Work out the finished part from the listing and answer in its coordinate system (mm). Face numbers are marked on the shaded views. A direction names the side the tool comes from. Coordinates: 2 decimals unless noted, no trailing zeros. Loops run counter-clockwise (first coordinate to the right, second up) from the corner with the lowest first, then second, coordinate; pieces in that order, holes last. Notation, with made-up numbers: (66, 18.25) -> (74, 18.25) arc R13 cw to (74, 36.25) -> close; hole circle Ø5 at (55, -23). An arc over 180 degrees is marked (long way). Use a Markdown table: item, result.
from build123d import *

# Parameters (mm, degrees)
SKETCH1_W           = 35
SKETCH1_H           = 25
BOSS_EXTRUDE1_DEPTH = 10
SKETCH2_R           = 3
CUT_EXTRUDE1_DEPTH  = 24.717082451
SKETCH3_W           = 18
SKETCH3_H           = 10
BOSS_EXTRUDE2_DEPTH = 20
SKETCH4_R           = 3
CUT_EXTRUDE2_DEPTH  = 38.831864876
FILLET2_R           = 15
FILLET3_R           = 2
CUT_EXTRUDE3_START  = -10
SKETCH5_R           = 3
CUT_EXTRUDE3_DEPTH  = 27.912057737
CUT_EXTRUDE4_START  = -10
CUT_EXTRUDE4_DEPTH  = 33.793107029


# Some blends are built 0.0001 mm under size
with BuildPart() as part:
    # Sketch1 → Boss-Extrude1 (new body)
    with BuildSketch(Plane.XY):
        Rectangle(SKETCH1_W, SKETCH1_H)
    extrude(amount=BOSS_EXTRUDE1_DEPTH)

    # Sketch2 → Cut-Extrude1 (cut, through all)
    with BuildSketch(Plane.XY.offset(10)):
        with Locations((-7.5, 2.5)):
            Circle(SKETCH2_R)
    extrude(amount=-CUT_EXTRUDE1_DEPTH, mode=Mode.SUBTRACT)

    # Sketch3 → Boss-Extrude2 (add)
    with BuildSketch(Plane.XY.offset(10)):
        with Locations((8.5, -7.5)):
            Rectangle(SKETCH3_W, SKETCH3_H)
    extrude(amount=BOSS_EXTRUDE2_DEPTH)

    # Sketch4 → Cut-Extrude2 (cut, through all)
    with BuildSketch(Plane(origin=(0, -2.5, 0), x_dir=(1, 0, 0), z_dir=(0, 1, 0))):
        with Locations(Location((8.5, -20, 0), (0, 0, 180))):
            Circle(SKETCH4_R)
    extrude(amount=-CUT_EXTRUDE2_DEPTH, mode=Mode.SUBTRACT)

    # Fillet2
    # the kernel refuses this fillet: 15 mm, written as the material it adds along each edge
    with BuildSketch(Plane(origin=(-0.5, -12.5, 10), x_dir=(-1, 0, 0), z_dir=(0, 1, 0))) as fillet2_piece_1:
        with BuildLine():
            CenterArc((FILLET2_R, FILLET2_R), FILLET2_R, 180, 90)
            Line((0, FILLET2_R), (0, 0))
            Line((0, 0), (FILLET2_R, 0))
        make_face()
    extrude(amount=10)
    with BuildSketch(Plane(origin=(-0.5, -2.5, 10), x_dir=(0, 1, 0), z_dir=(1, 0, 0))) as fillet2_piece_2_section:
        with BuildLine():
            CenterArc((FILLET2_R, FILLET2_R), FILLET2_R, 180, 90)
            Line((0, FILLET2_R), (0, 0))
            Line((0, 0), (FILLET2_R, 0))
        make_face()
    fillet2_piece_2 = extrude(amount=18, mode=Mode.PRIVATE)
    fillet2_piece_2 = fillet2_piece_2 - Plane(origin=(8.5, 1.000391612, 20), x_dir=(-1, 0, 0), z_dir=(0, 1, 0)) * Cylinder(3, 96, mode=Mode.PRIVATE)
    add(fillet2_piece_2)
    with BuildSketch(Plane(origin=(-0.5, -12.5, 10), x_dir=(-1, 0, 0), z_dir=(0, 1, 0))) as fillet2_piece_3a_section:
        with BuildLine():
            CenterArc((FILLET2_R, FILLET2_R), FILLET2_R, 180, 90)
            Line((0, FILLET2_R), (0, 0))
            Line((0, 0), (FILLET2_R, 0))
        make_face()
    fillet2_piece_3a = extrude(amount=47.5, mode=Mode.PRIVATE)
    fillet2_piece_3a = split(fillet2_piece_3a, bisect_by=Plane(origin=(-3.591955578, 12.5, 13.608814387), z_dir=(0, -1, 0)), keep=Keep.TOP, mode=Mode.PRIVATE)
    fillet2_piece_3a = fillet2_piece_3a - Plane(origin=(-7.5, 2.5, 13.608814387), x_dir=(1, 0, 0), z_dir=(0, 0, 1)) * Cylinder(3, 155, mode=Mode.PRIVATE)
    fillet2_piece_3a = split(fillet2_piece_3a, bisect_by=Plane(origin=(-3.591955578, -2.5, 13.608814387), z_dir=(0, 1, 0)), keep=Keep.TOP, mode=Mode.PRIVATE)
    with BuildSketch(Plane(origin=(-38, -2.5, 10), x_dir=(0, 1, 0), z_dir=(1, 0, 0))) as fillet2_piece_3b_section:
        with BuildLine():
            CenterArc((FILLET2_R, FILLET2_R), FILLET2_R, 180, 90)
            Line((0, FILLET2_R), (0, 0))
            Line((0, 0), (FILLET2_R, 0))
        make_face()
    fillet2_piece_3b = extrude(amount=55.5, mode=Mode.PRIVATE)
    fillet2_piece_3b = split(fillet2_piece_3b, bisect_by=Plane(origin=(-17.5, 8.593163462, 10.419487544), z_dir=(1, 0, 0)), keep=Keep.TOP, mode=Mode.PRIVATE)
    fillet2_piece_3b = fillet2_piece_3b - Plane(origin=(-7.5, 2.5, 10.419487544), x_dir=(1, 0, 0), z_dir=(0, 0, 1)) * Cylinder(3, 171, mode=Mode.PRIVATE)
    fillet2_piece_3b = split(fillet2_piece_3b, bisect_by=Plane(origin=(-0.5, 8.593163462, 10.419487544), z_dir=(-1, 0, 0)), keep=Keep.TOP, mode=Mode.PRIVATE)
    fillet2_piece_3 = fillet2_piece_3a & fillet2_piece_3b
    add(fillet2_piece_3)

    # Fillet3
    fillet3_edges = [part.edges().sort_by_distance(p)[0] for p in [
        (17.5, 0, 0),
        (-17.5, 0, 0),
        (-17.5, 0, 10),
        (-0.5, -7.5, 30),
        (17.5, -7.5, 30),
    ]]
    fillet(fillet3_edges, radius=FILLET3_R - 0.0001)  # a hair under: the kernel refuses the full size

    # Sketch5 → Cut-Extrude3 (cut, through all)
    with BuildSketch(Plane(origin=(0, 0, 0), x_dir=(-1, 0, 0), z_dir=(0, 0, -1)).offset(CUT_EXTRUDE3_START)):
        Polygon((2.5, 5.386751346), (2.5, -0.386751346), (7.5, -3.273502692), (12.5, -0.386751346), (12.5, 5.386751346), (7.5, 8.273502692), align=None)
        with Locations(Location((7.5, 2.5, 0), (0, 0, 180))):
            Circle(SKETCH5_R, mode=Mode.SUBTRACT)
    extrude(amount=-CUT_EXTRUDE3_DEPTH, mode=Mode.SUBTRACT)

    # Sketch6 → Cut-Extrude4 (cut, through all)
    with BuildSketch(Plane.XZ.offset(12.5).offset(CUT_EXTRUDE4_START)):
        Polygon((8.5, 14.111027254), (13.6, 17.055513627), (13.6, 22.944486373), (8.5, 25.888972746), (3.4, 22.944486373), (3.4, 17.055513627), align=None)
    extrude(amount=-CUT_EXTRUDE4_DEPTH, mode=Mode.SUBTRACT)


solid = part.part
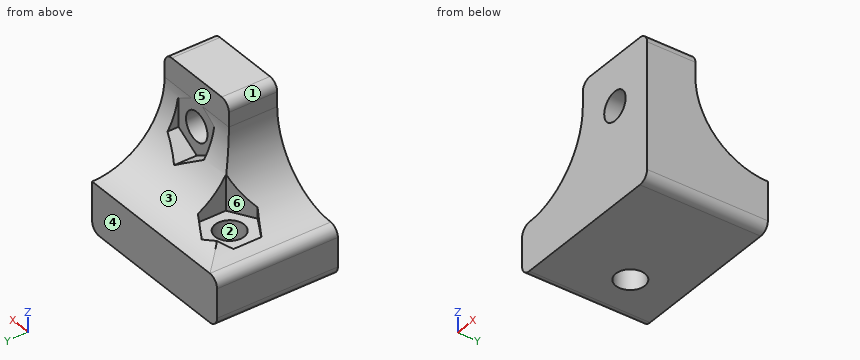
Q1. Determine the mould class of the marked faces 1, 2 and 3 for opening direction Y: pulls with the +Y half, pulls with the -Y half, needs draft (parallel to the pull), parting line crosses it, or undercut.
Solved:
| item | result |
|---|---|
| face 1 | needs draft |
| face 2 | undercut |
| face 3 | pulls with the +Y half |
Q2. For the marked faces 4, 5 and 6, determine the directions among +Z, -Z, +X, -X, +Y, -Y from which every point of the face is accessible in a straight line to the end or side of a thin tool.
Solved:
| item | result |
|---|---|
| face 4 | +Z, -Z, +X, -X, +Y |
| face 5 | +Y |
| face 6 | +Z |
Q3. Section C-C on z = 7.5 is taken. Determine the outline of the cut face in (x, y).
Solved:
| item | result |
|---|---|
| outline | (-17.5, -12.5) -> (17.5, -12.5) -> (17.5, 12.5) -> (-17.5, 12.5) -> close; hole circle Ø6 at (-7.5, 2.5) |
Q4. Given pin 1 Ø17.5 at (x, z) = (4.5, 24.5) entering from +Y; pin 2 Ø1.5 at (x, y) = (-11, 5.5) entering from +Z; pin 3 Ø9.5 at (x, z) = (8.5, 20) entering from +Y; pin 4 Ø3.5 at (x, y) = (-7.5, 2.5) entering from +Z, each flat-ended and moving along its own axis, determine where each tip first touches the part or whether it passes through.
Solved:
| item | result |
|---|---|
| pin 1 | y = 0.69 |
| pin 2 | z = 10.69 |
| pin 3 | y = -2.5 |
| pin 4 | through |
Q5. Section A-A on z = 20 is taken. Determine the outline of the cut face in (x, y), and give its area (3 significant figures).
Solved:
| item | result |
|---|---|
| outline | (-1.36, -12.5) -> (5.5, -12.5) -> (5.5, -2.5) -> (3.4, -2.5) -> (3.4, -1.64) -> (-1.36, -1.64) -> close; (11.5, -12.5) -> (17.5, -12.5) -> (17.5, -1.64) -> (13.6, -1.64) -> (13.6, -2.5) -> (11.5, -2.5) -> close |
| area | 136 mm² |
Q6. Consider line 1 (X direction, y = 2.5, z = 4.75); line 2 (Y direction, x = -7.5, z = 4); line 3 (Z direction, x = 9, y = -7.5). Determine where each line is inside the solid, lowest interval first. Write a range as [from, to].
Solved:
| item | result |
|---|---|
| line 1 | [-17.5, -10.5], [-4.5, 17.5] |
| line 2 | [-12.5, -0.5], [5.5, 12.5] |
| line 3 | [0, 17.04], [22.96, 30] |
